Here's the drawing with two shaded views (mm, measured from the low corner). I have some questions. A direction names the side the tool comes from. Coordinates: 2 decimals unless noted, no trailing zeros. Loops run counter-clockwise (first coordinate to the right, second up) from the corner with the lowest first, then second, coordinate; pieces in that order, holes last.
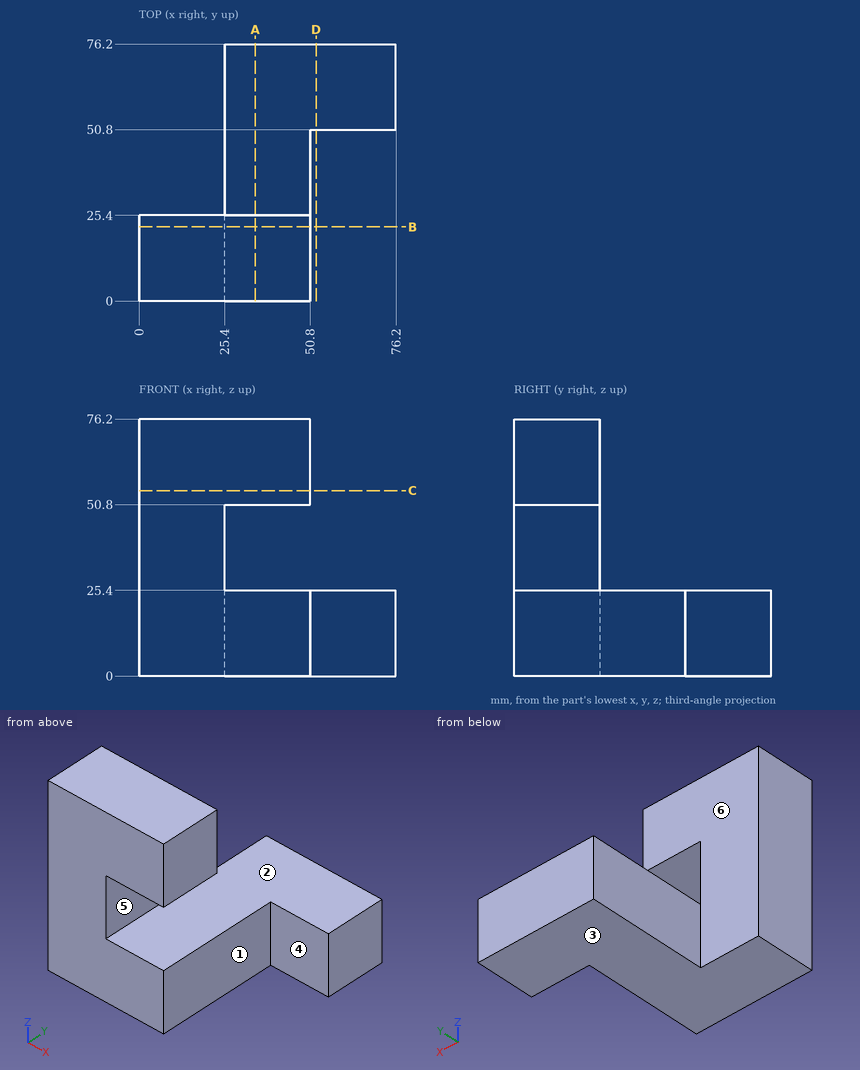
(1) If we mould it in two halves opening along Z, with no side actions, what happens to the marked faces 1, 2 and 3? For each: released by +Z, released by -Z, zero draft, split by the parting line, or undercut.
Check values:
face 1: zero draft
face 2: undercut
face 3: released by -Z
(2) I want a section at D-D on x = 52.5. Write out the boundary of the cut face in (y, z).
Check values:
outline: (50.8, 0) - (76.2, 0) - (76.2, 25.4) - (50.8, 25.4) - close
(3) I'm going to push flat-ended pins straight in: pin 1 (5 mm diameter, centred on x = 23, z = 44, fed in from +Y); pin 2 (12.5 mm diameter, centred on y = 50.5, z = 9, fed in from -X); pin 3 (4 mm diameter, centred on y = 30, z = 12, fed in from +X); pin 4 (20.5 mm diameter, centred on x = 57.5, z = 19, fed in from -Y). Where does each tip first touch, or does it pass through?
Check values:
pin 1: stops at y = 25.4
pin 2: stops at x = 25.4
pin 3: stops at x = 50.8
pin 4: stops at y = 0
(4) I want a section at B-B on y = 22. Write out the boundary of the cut face in (x, z).
Check values:
outline: (0, 0) - (50.8, 0) - (50.8, 25.4) - (25.4, 25.4) - (25.4, 50.8) - (50.8, 50.8) - (50.8, 76.2) - (0, 76.2) - close
(5) If I drill on probe 1 along Z at (x, y) = (47, 12.5); probe 2 along Z at (x, y) = (49, 66.5); probe 3 along X at (y, z) = (58, 23), over which ranges is the centre line in solid material (lowest first)?
Check values:
probe 1: z = 0 to 25.4, 50.8 to 76.2
probe 2: z = 0 to 25.4
probe 3: x = 25.4 to 76.2
(6) Which directions (+Z, -Z, +X, -X, +Y, -Y) give clear straight access to the entire face, cutting with the end or side of a thin tool? Please do the marked faces 4, 5 and 6.
Check values:
face 4: +Z, -Z, +X, -Y
face 5: +X, +Y, -Y
face 6: +Z, -X, +Y
(7) I want a section at A-A on x = 34.5. Write out the boundary of the cut face in (y, z).
Check values:
outline: (0, 0) - (76.2, 0) - (76.2, 25.4) - (0, 25.4) - close; (0, 50.8) - (25.4, 50.8) - (25.4, 76.2) - (0, 76.2) - close
(8) I want a section at C-C on z = 55. Write out the boundary of the cut face in (x, y).
Check values:
outline: (0, 0) - (50.8, 0) - (50.8, 25.4) - (0, 25.4) - close
